Geometry: final body of the model. Coordinates: model frame, mm. Give positions to 0.01 mm unless a question says otherwise; leave off trailing zeros. Loops run counter-clockwise (first coordinate to the right, second up) from the corner with the lowest first, then second, coordinate; pieces in that order, holes last.
1. First-contact query: P1, Ø1.5, axis at x = 32.5, y = 1.5, coming from the +Z side; P2, Ø10, axis at x = 26.162, z = -14.224, coming from the +Y side; P3, Ø2.5, axis at y = 3.5, z = 28, coming from the +X side; P4, Ø2.5, axis at x = -60, y = 1.5, coming from the +Z side. Flat tips, straight axial feed; report the tip coordinate or a pass-through.
2. Section B-B, the plane x = -30. Output: boundary loops of the cut face in (y, z), then the cut area to 3 significant figures.
3. Section A-A, the plane z = -8. Output: boundary loops of the cut face in (x, y), then the cut area to 3 significant figures.
4. Section C-C, the plane z = 2. Output: boundary loops of the cut face in (x, y), then the cut area to 3 significant figures.
5. Section D-D, the plane y = 1.1. State how many separate pieces and enclosed holes the cut face has, then the cut area to 3 significant figures.
6. Material intervals for line 1 along X through (y, z) = (2.65, 0); line 2 along Z through (x, y) = (28, 4.05); line 3 along X through (y, z) = (1.95, -19), sorted ascending.
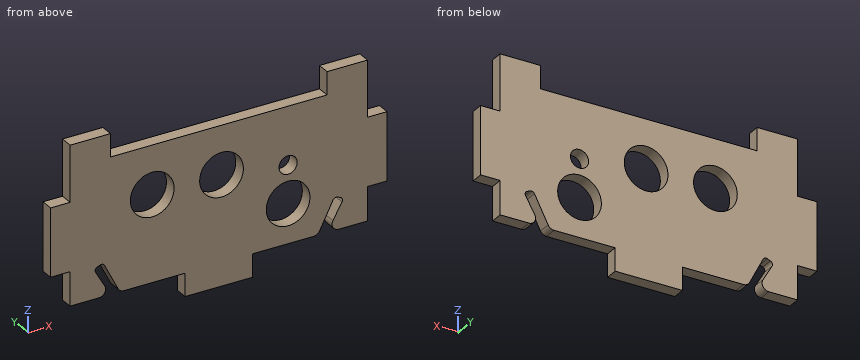
from build123d import *

# Parameters (mm, degrees)
BOSS_EXTRUDE1_DEPTH = 4.826
FILLET1_R           = 1.27
SKETCH2_R           = 8.255
SKETCH2_R_2         = 3.429
CUT_EXTRUDE1_DEPTH  = 75.015290562
FILLET2_R           = 2.54


with BuildPart() as part:
    # Sketch1 → Boss-Extrude1 (new body)
    with BuildSketch(Plane(origin=(0, 0, 0), x_dir=(1, 0, 0), z_dir=(0, 1, 0))):
        Polygon((-56.134, 29.083), (-40.894, 29.083), (-47.241885042, 18.083256572), (-43.685885042, 16.624574128), (-37.338, 29.083), (-12.7, 29.083), (-12.7, 37.719), (12.7, 37.719), (12.7, 29.083), (37.338, 29.083), (43.685885042, 16.624574128), (47.241885042, 18.083256572), (40.894, 29.083), (56.134, 29.083), (56.134, 16.383), (63.5, 16.383), (63.5, -9.230617291), (56.134, -9.230617291), (56.134, -29.083), (56.134, -30.353), (40.894, -30.353), (40.894, -21.717), (-40.894, -21.717), (-40.894, -30.353), (-56.134, -30.353), (-56.134, -29.083), (-56.134, -9.230617291), (-63.5, -9.230617291), (-63.5, 16.383), (-56.134, 16.383), align=None)
    extrude(amount=BOSS_EXTRUDE1_DEPTH)

    # Fillet1
    fillet1_edges = [part.edges().sort_by_distance(p)[0] for p in [
        (-47.241885042, 2.413, -18.083256572),
        (-43.685885042, 2.413, -16.624574128),
        (43.685885042, 2.413, -16.624574128),
        (47.241885042, 2.413, -18.083256572),
    ]]
    fillet(fillet1_edges, radius=FILLET1_R)

    # Sketch2 → Cut-Extrude1 (cut, through all)
    with BuildSketch(Plane(origin=(0, 4.826, 0), x_dir=(1, 0, 0), z_dir=(0, 1, 0))):
        with Locations(Location((26.162, 14.224, 0), (0, 0, 270))):
            Circle(SKETCH2_R)
        with Locations(Location((26.162, 0, 0), (0, 0, 270))):
            Circle(SKETCH2_R_2)
        with Locations(Location((-25.146, -3.429, 0), (0, 0, 270))):
            Circle(SKETCH2_R)
        with Locations(Location((1.016, -3.429, 0), (0, 0, 270))):
            Circle(SKETCH2_R)
    extrude(amount=-CUT_EXTRUDE1_DEPTH, mode=Mode.SUBTRACT)

    # Fillet2
    fillet2_edges = [part.edges().sort_by_distance(p)[0] for p in [
        (-40.894, 2.413, -29.083),
        (-37.338, 2.413, -29.083),
        (37.338, 2.413, -29.083),
        (40.894, 2.413, -29.083),
    ]]
    fillet(fillet2_edges, radius=FILLET2_R)


solid = part.part
Answers below:
1. P1: stops at z = 21.72
1. P2: passes through
1. P3: stops at x = 56.13
1. P4: stops at z = 9.23
2. outline: (0, -29.08) - (4.83, -29.08) - (4.83, -3.25) - (0, -3.25) - close; (0, 10.11) - (4.83, 10.11) - (4.83, 21.72) - (0, 21.72) - close
2. area: 181 mm2
3. outline: (-63.5, 0) - (20.74, 0) - (20.74, 4.83) - (-63.5, 4.83) - close; (31.58, 0) - (63.5, 0) - (63.5, 4.83) - (31.58, 4.83) - close
3. area: 561 mm2
4. outline: (-63.5, 0) - (-33.28, 0) - (-33.28, 4.83) - (-63.5, 4.83) - close; (-17.02, 0) - (-7.11, 0) - (-7.11, 4.83) - (-17.02, 4.83) - close; (9.15, 0) - (23.38, 0) - (23.38, 4.83) - (9.15, 4.83) - close; (28.95, 0) - (63.5, 0) - (63.5, 4.83) - (28.95, 4.83) - close
4. area: 429 mm2
5. separate pieces: 1
5. enclosed holes: 4
5. area: 5,780 mm2
6. line 1: x = -63.5 to -32.66, -17.64 to -6.49, 8.53 to 22.73, 29.59 to 63.5
6. line 2: z = -29.08 to -22.27, -6.18 to -2.89, 2.89 to 21.72
6. line 3: x = -56.13 to -46.65, -42.48 to 19.43, 32.9 to 42.48, 46.65 to 56.13
